Geometry check sheet. Reference: the model listing, model coordinates, mm. A direction names the side the tool comes from. Coordinates: 2 decimals unless noted, no trailing zeros. Loops run counter-clockwise (first coordinate to the right, second up) from the corner with the lowest first, then second, coordinate; pieces in that order, holes last. Notation, with made-up numbers: (59, 49.25) - (102, 49.25) arc R25 ccw to (102, 61.25) - close; hole circle Ø7 at (10.25, -26.75). An arc over 180 degrees is marked (long way). One line per item, written item: value.
from build123d import *

# Parameters (mm, degrees)
BOSS_EXTRUDE1_DEPTH = 10
SKETCH2_R           = 1.5
CUT_EXTRUDE1_DEPTH  = 25.5


with BuildPart() as part:
    # Sketch1 → Boss-Extrude1 (new body)
    with BuildSketch(Plane(origin=(0, 0, 0), x_dir=(1, 0, 0), z_dir=(0, 1, 0))):
        with BuildLine():
            Line((-0.5, 37.994564575), (-0.5, 22.994564575))
            ThreePointArc((-0.5, 22.994564575), (0, -23), (0.5, 22.994564575))
            Line((0.5, 22.994564575), (0.5, 37.994564575))
            Line((0.5, 37.994564575), (1, 37.994564575))
            Line((1, 37.994564575), (1, 23.478713764))
            ThreePointArc((1, 23.478713764), (0, -23.5), (-1, 23.478713764))
            Line((-1, 23.478713764), (-1, 37.994564575))
            Line((-1, 37.994564575), (-0.5, 37.994564575))
        make_face()
    extrude(amount=BOSS_EXTRUDE1_DEPTH)

    # Sketch2 → Cut-Extrude1 (cut, through all)
    with BuildSketch(Plane(origin=(1, 0, 0), x_dir=(0, 0, -1), z_dir=(1, 0, 0))):
        with Locations((33.478713764, 4.782975317)):
            Circle(SKETCH2_R)
    extrude(amount=-CUT_EXTRUDE1_DEPTH, mode=Mode.SUBTRACT)


solid = part.part
(1) Go/stop test with flat-tipped pins: pin 1 Ø6 at (y, z) = (1.5, 7) entering from -X; pin 2 Ø5 at (y, z) = (3, -33.5) entering from -X; pin 3 Ø6 at (x, y) = (-16.5, 7.5) entering from -Z; pin 4 Ø10 at (x, z) = (15, -12.5) entering from -Y. Record where each tip stops, or that it passes through.
Reply:
pin 1: x = -23.16
pin 2: x = -1
pin 3: z = -19.24
pin 4: y = 0
(2) Cross-section at C-C on y = 8.5. Record the cut outline in (x, z).
Reply:
outline: (-1, -37.99) - (-0.5, -37.99) - (-0.5, -22.99) arc R23 cw (long way) to (0.5, -22.99) - (0.5, -37.99) - (1, -37.99) - (1, -23.48) arc R23.5 ccw (long way) to (-1, -23.48) - close
(3) Material ranges on probe 1 along X at (y, z) = (6, -27.5); probe 2 along Z at (x, y) = (-16, 6.25); probe 3 along Z at (x, y) = (21, 4.5), recorded low to high. Write a range as from..to.
Reply:
probe 1: -1..-0.5, 0.5..1
probe 2: -17.21..-16.52, 16.52..17.21
probe 3: -10.55..-9.38, 9.38..10.55
(4) Access from +Z, -Z, +X, -X, +Y, -Y to the whole of each face (thin tool, end or side, straight path). Record for faces 4 (the face through (-0.5, 5, -31)), 5 (the face through (-1, 5, -31)), 6 (the face through (-6.9, 0, 22.2)).
Reply:
face 4: -Z, +Y, -Y
face 5: -Z, -X, +Y, -Y
face 6: +Z, -Z, +X, -X, -Y
(5) Cross-section at D-D on y = 4. Record the cut outline in (x, z), and give its area (3 significant figures).
Reply:
outline: (-1, -37.99) - (-0.5, -37.99) - (-0.5, -34.76) - (-1, -34.76) - close; (-1, -32.2) - (-0.5, -32.2) - (-0.5, -22.99) arc R23 cw (long way) to (0.5, -22.99) - (0.5, -32.2) - (1, -32.2) - (1, -23.48) arc R23.5 ccw (long way) to (-1, -23.48) - close; (0.5, -37.99) - (1, -37.99) - (1, -34.76) - (0.5, -34.76) - close
area: 84.5 mm2
(6) Release check for a two-part mould opening along Z. For faces 1 (the face through (0.75, 3.87, -32.29)), 2 (the face through (1.019, 4.93, 23.478)), 3 (the face through (1, 5, -31)) record: pulls with the +Z half, pulls with the -Z half, needs draft (parallel to the pull), parting line crosses it, or undercut.
Reply:
face 1: undercut
face 2: parting line crosses it
face 3: needs draft
(7) Cross-section at A-A on z = 0. Record the cut outline in (x, y), and give its area (3 significant figures).
Reply:
outline: (-23.5, 0) - (-23, 0) - (-23, 10) - (-23.5, 10) - close; (23, 0) - (23.5, 0) - (23.5, 10) - (23, 10) - close
area: 10.0 mm2
(8) Cross-section at B-B on x = -15.5. Record the cut outline in (y, z), and give its area (3 significant figures).
Reply:
outline: (0, -17.66) - (10, -17.66) - (10, -16.99) - (0, -16.99) - close; (0, 16.99) - (10, 16.99) - (10, 17.66) - (0, 17.66) - close
area: 13.4 mm2
